The model under review builds one solid part; all positions refer to its coordinate system, in mm. Face numbers are marked on the shaded views. A direction names the side the tool comes from. Round coordinates to 2 decimals unless told otherwise and drop trailing zeros. Order: outer loops, then holes, each group sorted by start corner. A loop starts at its lowest first (then second) coordinate and runs counter-clockwise, first axis right, second up. Notation, with made-up numbers: M 37.25,7.5 L 86.25,7.5 A26 cw 86.25,25.5 Z; hole C -17,19.25 d9. An arc over 180 degrees is marked long. Answer as a JSON object with one key per item and string values. Group by question number.
1) The part is to be moulded in two halves that separate along Y. For the marked faces 1, 2, 3 and 4, say which applies: +Y half, -Y half, draft (parallel to the pull), parting line (faces both ways), or undercut.
2) Insertion check: pin 1 Ø5 at (x, z) = (0, 55.5) entering from +Y; pin 2 Ø13 at (x, z) = (3.5, 56) entering from +Y; pin 3 Ø11 at (y, z) = (9, 37) entering from -X; pin 4 Ø2.5 at (x, z) = (0, 40.1) entering from +Y. Each pin has a flat end and moves straight along its axis. Give the tip position at first contact, or say it passes through.
3) To check wall thickness, follow line 1 (Z direction, x = 0, y = 14.8); line 2 (X direction, y = 10.75, z = 0); line 3 (X direction, y = 1.5, z = 41). State the ranges of each line that lie inside material, in increasing order.
4) For the marked faces 5, 6 and 7, list the 3-axis set-ups (+Z, -Z, +X, -X, +Y, -Y) from which the entire face can be reached by the end or side of a thin tool; tool diameter is ignored.
5) Consider section C-C, the plane y = 8.75. Write out the cut boundary in (x, z).
6) Consider section B-B, the plane z = 40.1. Write out the cut boundary in (x, y).
7) Consider section A-A, the plane x = 0. Count the separate pieces of the cut face and the enclosed holes in it, then the cut area to 3 significant figures.
8) Consider section D-D, the plane z = 0. Write out the cut boundary in (x, y), then the cut area to 3 significant figures.
```python
from build123d import *

# Parameters (mm, degrees)
ESQUISSE1_R                    = 32.5
BOSS_EXTRU_1_DEPTH             = 4
ESQUISSE2_R                    = 32.5
ESQUISSE2_R_2                  = 23
BOSS_EXTRU_2_DEPTH             = 10
ESQUISSE4_R                    = 30.8
ESQUISSE4_R_2                  = 28.8
BOSS_EXTRU_4_DEPTH             = 7
BOSS_EXTRU_5_DEPTH             = 35
BOSS_EXTRU_5_DIRECTION_2_REACH = 67
ESQUISSE6_R                    = 2
ENL_V_MAT_EXTRU_1_DEPTH        = 5
CHANFREIN1_SIZE                = 3
ENL_V_MAT_EXTRU_2_REACH        = 67
ESQUISSE8_W                    = 4
ESQUISSE8_H                    = 8


with BuildPart() as part:
    # Esquisse1 → Boss.-Extru.1 (new body)
    with BuildSketch(Plane(origin=(0, 0, 0), x_dir=(1, 0, 0), z_dir=(0, 1, 0))):
        Circle(ESQUISSE1_R)
    extrude(amount=BOSS_EXTRU_1_DEPTH)

    # Esquisse2 → Boss.-Extru.2 (add)
    with BuildSketch(Plane(origin=(0, 4, 0), x_dir=(1, 0, 0), z_dir=(0, 1, 0))):
        Circle(ESQUISSE2_R)
        Circle(ESQUISSE2_R_2, mode=Mode.SUBTRACT)
    extrude(amount=BOSS_EXTRU_2_DEPTH)

    # Esquisse4 → Boss.-Extru.4 (add)
    with BuildSketch(Plane(origin=(0, 14, 0), x_dir=(1, 0, 0), z_dir=(0, 1, 0))):
        Circle(ESQUISSE4_R)
        Circle(ESQUISSE4_R_2, mode=Mode.SUBTRACT)
    extrude(amount=BOSS_EXTRU_4_DEPTH)

    # Esquisse5 → Boss.-Extru.5 (add)
    with BuildSketch(Plane.XY.offset(32.5)):
        Polygon((13, 18.5), (-13, 18.5), (-13, 0), (-10.5, 0), (-10.5, 14), (10.5, 14), (10.5, 0), (13, 0), align=None)
    extrude(amount=BOSS_EXTRU_5_DEPTH)

    # Esquisse5 → Boss.-Extru.5 direction 2 (add, up to next)
    with BuildSketch(Plane.XY.offset(32.5), mode=Mode.PRIVATE) as boss_extru_5_direction_2_sk1:
        Polygon((13, 18.5), (-13, 18.5), (-13, 0), (-10.5, 0), (-10.5, 14), (10.5, 14), (10.5, 0), (13, 0), align=None)
    boss_extru_5_direction_2_tool1 = extrude(boss_extru_5_direction_2_sk1.sketch, amount=-BOSS_EXTRU_5_DIRECTION_2_REACH, mode=Mode.PRIVATE) - part.part
    add(boss_extru_5_direction_2_tool1.solids().sort_by_distance((0, 18.1809, 32.5))[0])

    # Esquisse6 → Enlèv. mat.-Extru.1 (cut)
    with BuildSketch(Plane(origin=(0, 18.5, 0), x_dir=(1, 0, 0), z_dir=(0, 1, 0))):
        with Locations((0, -55.5)):
            Circle(ESQUISSE6_R)
        with Locations((0, -40.1)):
            Circle(ESQUISSE6_R)
    extrude(amount=-ENL_V_MAT_EXTRU_1_DEPTH, mode=Mode.SUBTRACT)

    # Chanfrein1
    chanfrein1_edges = [part.edges().sort_by_distance(p)[0] for p in [
        (-2, 18.5, 55.5),
        (-2, 18.5, 40.1),
    ]]
    chamfer(chanfrein1_edges, length=CHANFREIN1_SIZE)

    # Esquisse8 → Enlèv. mat.-Extru.2 (cut, up to next)
    with BuildSketch(Plane.XY.offset(32.5), mode=Mode.PRIVATE) as enl_v_mat_extru_2_sk1:
        with Locations((-8.5, 8)):
            Rectangle(ESQUISSE8_W, ESQUISSE8_H)
    enl_v_mat_extru_2_tool1 = extrude(enl_v_mat_extru_2_sk1.sketch, amount=-ENL_V_MAT_EXTRU_2_REACH, mode=Mode.PRIVATE) & part.part
    add(enl_v_mat_extru_2_tool1.solids().sort_by_distance((-8.5, 8, 32.5))[0], mode=Mode.SUBTRACT)
    # Esquisse8 → Enlèv. mat.-Extru.2 (cut, up to next)
    with BuildSketch(Plane.XY.offset(32.5), mode=Mode.PRIVATE) as enl_v_mat_extru_2_sk2:
        with Locations((8.5, 8)):
            Rectangle(ESQUISSE8_W, ESQUISSE8_H)
    enl_v_mat_extru_2_tool2 = extrude(enl_v_mat_extru_2_sk2.sketch, amount=-ENL_V_MAT_EXTRU_2_REACH, mode=Mode.PRIVATE) & part.part
    add(enl_v_mat_extru_2_tool2.solids().sort_by_distance((8.5, 8, 32.5))[0], mode=Mode.SUBTRACT)


solid = part.part
```
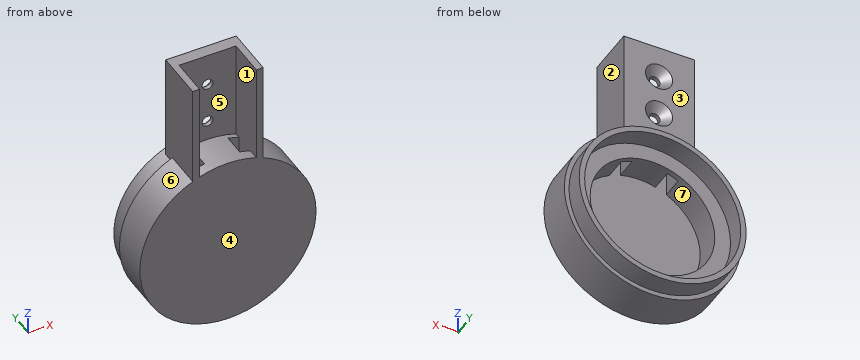
Results list:
{
 "1": {"face 1": "undercut", "face 2": "draft", "face 3": "+Y half", "face 4": "-Y half"},
 "2": {"pin 1": "y = 16", "pin 2": "y = 18.5", "pin 3": "x = -13", "pin 4": "through"},
 "3": {"line 1": "-30.8 to -28.8, 28.8 to 38.1, 42.1 to 53.5, 57.5 to 67.5", "line 2": "-32.5 to -23, 23 to 32.5", "line 3": "-13 to -10.5, 10.5 to 13"},
 "4": {"face 5": "+Z, -Y", "face 6": "+Y, -Y", "face 7": "+Y"},
 "5": {"outline": "M -13,29.79 A32.5 ccw long 13,29.79 L 13,67.5 L 10.5,67.5 L 10.5,20.46 A23 cw long -10.5,20.46 L -10.5,67.5 L -13,67.5 Z; M -6.5,22.06 A23 cw 6.5,22.06 L 6.5,31.84 A32.5 ccw -6.5,31.84 Z"},
 "6": {"outline": "M -13,0 L -10.5,0 L -10.5,14 L -2,14 L -2,15.5 L -5,18.5 L -13,18.5 Z; M 2,14 L 10.5,14 L 10.5,0 L 13,0 L 13,18.5 L 5,18.5 L 2,15.5 Z"},
 "7": {"separate pieces": "3", "enclosed holes": "0", "area": "589 mm^2"},
 "8": {"outline": "M -32.5,0 L 32.5,0 L 32.5,14 L 30.8,14 L 30.8,21 L 28.8,21 L 28.8,14 L 23,14 L 23,4 L -23,4 L -23,14 L -28.8,14 L -28.8,21 L -30.8,21 L -30.8,14 L -32.5,14 Z", "area": "478 mm^2"}
}
